```python
from build123d import *

# Parameters (mm, degrees)
PAD_DEPTH       = 42
PAD001_DEPTH    = 2
POCKET_DEPTH    = 2
PAD002_DEPTH    = 4
FILLET_R        = 5
SKETCH004_R     = 1.25
SKETCH004_W     = 7
SKETCH004_H     = 7
PAD003_DEPTH    = 6
FILLET001_R     = 4
SKETCH005_R     = 7.5
POCKET001_DEPTH = 1
SKETCH006_R     = 5
POCKET002_DEPTH = 1
SKETCH008_R     = 1.5
POCKET004_DEPTH = 5
CHAMFER_SIZE    = 1


with BuildPart() as part:
    # Sketch → Pad (new body)
    with BuildSketch(Plane.XY):
        Polygon((-17.5, 4), (-17.5, 7), (-24, 7), (-24, -3), (-19.5, -19), (19.5, -19), (24, -3), (24, 7), (17.5, 7), (17.5, 4), (21, 4), (21, 0), (16.5, 0), (16.5, -17), (-16.5, -17), (-16.5, 0), (-21, 0), (-21, 4), align=None)
    extrude(amount=PAD_DEPTH)

    # Sketch001 (on Face19 of Pad) → Pad001 (join)
    with BuildSketch(Plane(origin=(0, 0, 0), x_dir=(1, 0, 0), z_dir=(0, 0, -1))):
        Polygon((-19.5, 19), (19.5, 19), (24, 3), (24, -7), (-24, -7), (-24, 3), align=None)
    extrude(amount=PAD001_DEPTH)

    # Sketch002 (on Face18 of Pad001) → Pocket (cut)
    with BuildSketch(Plane.XZ.offset(19)):
        Polygon((-4, 31.071797), (0, 38), (4, 31.071797), align=None)
        Polygon((-2.828427, 15), (0, 17.828427), (2.828427, 15), (0, 12.171573), align=None)
    extrude(amount=-POCKET_DEPTH, mode=Mode.SUBTRACT)

    # Sketch003 (on Face12 of Pocket) → Pad002 (join)
    with BuildSketch(Plane(origin=(0, 0, 0), x_dir=(-1, 0, 0), z_dir=(0, 1, 0))):
        Polygon((-21, 29), (-21, 25), (-19.5, 27), align=None)
        Polygon((21, 29), (21, 25), (19.5, 27), align=None)
    extrude(amount=PAD002_DEPTH)

    # Fillet
    fillet_edges = [part.edges().sort_by_distance(p)[0] for p in [
        (-24, -3, 21),
        (-19.5, -19, 21),
        (19.5, -19, 21),
        (24, -3, 21),
    ]]
    fillet(fillet_edges, radius=FILLET_R)

    # Sketch004 (on Face16 of Fillet) → Pad003 (join)
    with BuildSketch(Plane(origin=(0, -17, 0), x_dir=(-1, 0, 0), z_dir=(0, 1, 0))):
        Polygon((-16.5, 42), (-9.5, 42), (-9.5, 37), (-16.5, 30), align=None)
        with Locations((-12.7, 38.56)):
            Circle(SKETCH004_R, mode=Mode.SUBTRACT)
        Polygon((16.5, 42), (9.5, 42), (9.5, 37), (16.5, 30), align=None)
        with Locations((12.7, 38.56)):
            Circle(SKETCH004_R, mode=Mode.SUBTRACT)
        with Locations((-13, 3.5)):
            Rectangle(SKETCH004_W, SKETCH004_H)
        with Locations((-12.7, 3)):
            Circle(SKETCH004_R, mode=Mode.SUBTRACT)
        with Locations((13, 3.5)):
            Rectangle(SKETCH004_W, SKETCH004_H)
        with Locations((12.7, 3)):
            Circle(SKETCH004_R, mode=Mode.SUBTRACT)
    extrude(amount=PAD003_DEPTH)

    # Fillet001
    fillet001_edges = [part.edges().sort_by_distance(p)[0] for p in [
        (9.5, -14, 37),
        (9.5, -14, 7),
        (-9.5, -14, 7),
        (-9.5, -14, 37),
    ]]
    fillet(fillet001_edges, radius=FILLET001_R)

    # Sketch005 (on Face7 of Fillet001) → Pocket001 (cut)
    with BuildSketch(Plane.XY):
        with Locations((0, -2)):
            Circle(SKETCH005_R)
    extrude(amount=-POCKET001_DEPTH, mode=Mode.SUBTRACT)

    # Sketch006 (on Face62 of Pocket001) → Pocket002 (cut)
    with BuildSketch(Plane.XY.offset(-1)):
        with Locations((0, -2)):
            Circle(SKETCH006_R)
    extrude(amount=-POCKET002_DEPTH, mode=Mode.SUBTRACT)

    # Sketch008 (on Face12 of Pocket002) → Pocket004 (cut)
    with BuildSketch(Plane.XY.offset(42)):
        with Locations((-20, -4)):
            Circle(SKETCH008_R)
        with Locations((20, -4)):
            Circle(SKETCH008_R)
    extrude(amount=-POCKET004_DEPTH, mode=Mode.SUBTRACT)

    # Chamfer
    chamfer_edges = [part.edges().sort_by_distance(p)[0] for p in [
        (0, -19, -2),
        (0, 7, -2),
    ]]
    chamfer(chamfer_edges, length=CHAMFER_SIZE)


solid = part.part
```
Part model, mm, in its own coordinate system. A direction names the side the tool comes from. Round coordinates to 2 decimals unless told otherwise and drop trailing zeros. Loops run counter-clockwise (first coordinate to the right, second up) from the corner with the lowest first, then second, coordinate; pieces in that order, holes last. Notation, with made-up numbers: (5.25, 23.5) -> (63.25, 23.5) arc R19 ccw to (63.25, 54.5) -> close; hole circle Ø7 at (1, 28.25). An arc over 180 degrees is marked (long way). Use one line per item in the form item = value. Start each with the question number.
Item 1: Band-saw the part on A-A (y = -12.5). List the corners of the cut face in (x, z).
Item 2: Drop flat-ended pins along their axis: pin 1 Ø3.5 at (y, z) = (-13, 40.5) entering from -X; pin 2 Ø4 at (y, z) = (-12, 29) entering from +X; pin 3 Ø3.5 at (x, z) = (11.5, 3) entering from +Y; pin 4 Ø8 at (x, z) = (-16.5, 17.5) entering from -Y. Give the stop position or say it passes through.
Item 3: Two-plate mould, pull along X, no slides. Class faces 1 (the cylindrical face through (-9.796, -13.958, 37.146)), 2 (the flat face through (0, -9, -2)), 3 (the conical face through (23.45, -2.933, -1.507)): released by +X, released by -X, zero draft, split by the parting line, or undercut.
Item 4: Band-saw the part on C-C (z = 17). List the corners of the cut face in (x, y).
Item 5: Band-saw the part on D-D (y = -16). Give the number of separate pieces and of enclosed holes in the cut face, plus the area to 3 significant figures.
Item 6: Band-saw the part on B-B (x = 1). List the corners of the cut face in (y, z).
Item 7: Tool access for faces 4 (the flat face through (17.5, 6, 21)), 5 (the flat face through (13.5, -14, 33)), 6 (the cylindrical face through (-7.493, -1.67, -0.493)), 7 (the flat face through (-2.028, -18.014, 34.487)): list every direction of +Z, -Z, +X, -X, +Y, -Y with a clear straight run to the whole face (end or side of a thin tool).
Item 8: Drill centre lines: line 1 along X through (y, z) = (2.5, 2); line 2 along X through (y, z) = (-1.25, 33); line 3 along Y through (x, z) = (20, 39). Where is each one in solid material? Low to high.
Data:
q1.outline = (-21.33, -1) -> (-20.29, -2) -> (20.29, -2) -> (21.33, -1) -> (21.33, 42) -> (9.5, 42) -> (9.5, 38.66) arc R4 ccw to (10.67, 35.83) -> (16.5, 30) -> (16.5, 7) -> (13.5, 7) arc R4 ccw to (9.5, 3) -> (9.5, 0) -> (-9.5, 0) -> (-9.5, 3) arc R4 ccw to (-13.5, 7) -> (-16.5, 7) -> (-16.5, 30) -> (-10.67, 35.83) arc R4 ccw to (-9.5, 38.66) -> (-9.5, 42) -> (-21.33, 42) -> close; hole circle Ø2.5 at (-12.7, 3); hole circle Ø2.5 at (-12.7, 38.56); hole circle Ø2.5 at (12.7, 3); hole circle Ø2.5 at (12.7, 38.56)
q2.pin_1 = -21.68
q2.pin_2 = 22.03
q2.pin_3 = -11
q2.pin_4 = -19
q3.face_1 = undercut
q3.face_2 = zero draft
q3.face_3 = released by +X
q4.outline = (-24, -2.31) arc R5 ccw to (-23.81, -3.66) -> (-20.53, -15.35) arc R5 ccw to (-15.71, -19) -> (-0.83, -19) -> (-0.83, -17) -> (-16.5, -17) -> (-16.5, 0) -> (-21, 0) -> (-21, 4) -> (-17.5, 4) -> (-17.5, 7) -> (-24, 7) -> close; (0.83, -19) -> (15.71, -19) arc R5 ccw to (20.53, -15.35) -> (23.81, -3.66) arc R5 ccw to (24, -2.31) -> (24, 7) -> (17.5, 7) -> (17.5, 4) -> (21, 4) -> (21, 0) -> (16.5, 0) -> (16.5, -17) -> (0.83, -17) -> close
q5.separate_pieces = 1
q5.enclosed_holes = 4
q5.area = 589 mm^2
q6.outline = (-19, -1) -> (-18, -2) -> (-6.9, -2) -> (-6.9, -1) -> (-9.43, -1) -> (-9.43, 0) -> (-17, 0) -> (-17, 13.17) -> (-19, 13.17) -> close; (-19, 16.83) -> (-17, 16.83) -> (-17, 31.07) -> (-19, 31.07) -> close; (-19, 36.27) -> (-17, 36.27) -> (-17, 42) -> (-19, 42) -> close; (2.9, -2) -> (6, -2) -> (7, -1) -> (7, 0) -> (5.43, 0) -> (5.43, -1) -> (2.9, -1) -> close
q7.face_4 = +Z, +Y
q7.face_5 = +Y
q7.face_6 = +Z
q7.face_7 = +Y, -Y
q8.line_1 = -24 to -21, 21 to 24
q8.line_2 = -24 to -16.5, 16.5 to 24
q8.line_3 = -16.57 to -5.5, -2.5 to 0, 4 to 7
